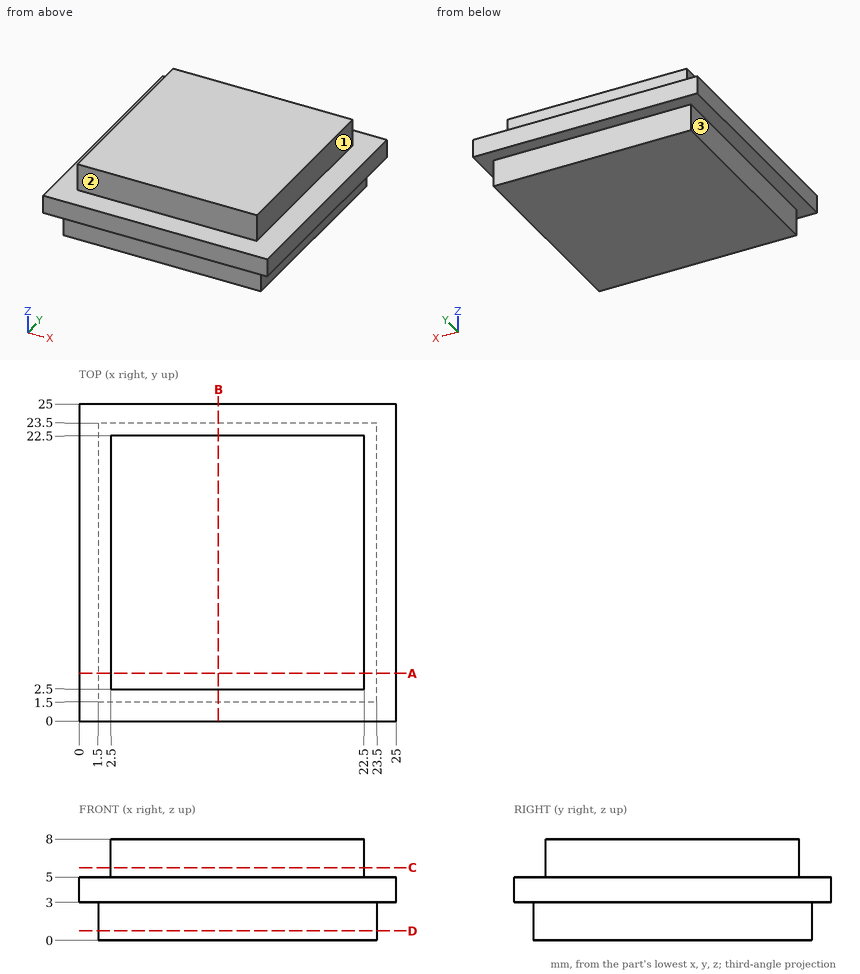
The drawing under review shows one solid part. Ordinate dimensions are in mm from its lowest x, y, z. A direction names the side the tool comes from. Coordinates: 2 decimals unless noted, no trailing zeros. Write each loop counter-clockwise with the first axis right and the second up, starting at its lowest first coordinate (ties: lowest second). Pieces come first, ordered by that corner, then holes. Notation, with made-up numbers: (-25.75, 21) -> (19.25, 21) arc R33 cw to (19.25, 60) -> close; hole circle Ø8 at (5.25, 80). An arc over 180 degrees is marked (long way). Write each question's results on one line, items separated by ' | '. Start each with the question number.
1) Consider section D-D (z = 0.75). Write out the cut boundary in (x, y).
2) Insertion check: pin 1 (0.9 mm diameter, centred on y = 16, z = 2, fed in from -X); pin 2 (0.9 mm diameter, centred on x = 9, z = 2, fed in from -Y); pin 3 (1.5 mm diameter, centred on x = 8, z = 2, fed in from +Y). Each pin has a flat end and moves straight along its axis. Give the tip position at first contact, or say it passes through.
3) Wall thickness on L1, parallel to Y at x = 3.5, z = 7.5; L2, parallel to X at y = 14.5, z = 1: over which ranges is each line inside the solid? List them lowest first. Write a range as [from, to].
4) Consider section C-C (z = 5.75). Write out the cut boundary in (x, y).
5) For the marked faces 1, 2 and 3, list the 3-axis set-ups (+Z, -Z, +X, -X, +Y, -Y) from which the entire face can be reached by the end or side of a thin tool; tool diameter is ignored.
6) Consider section A-A (y = 3.75). Write out the cut boundary in (x, z).
Geometry says:
1) outline: (1.5, 1.5) -> (23.5, 1.5) -> (23.5, 23.5) -> (1.5, 23.5) -> close
2) pin 1: x = 1.5 | pin 2: y = 1.5 | pin 3: y = 23.5
3) L1: [2.5, 22.5] | L2: [1.5, 23.5]
4) outline: (2.5, 2.5) -> (22.5, 2.5) -> (22.5, 22.5) -> (2.5, 22.5) -> close
5) face 1: +Z, +X, +Y, -Y | face 2: +Z, +X, -X, -Y | face 3: -Z, -X, +Y, -Y
6) outline: (0, 3) -> (1.5, 3) -> (1.5, 0) -> (23.5, 0) -> (23.5, 3) -> (25, 3) -> (25, 5) -> (22.5, 5) -> (22.5, 8) -> (2.5, 8) -> (2.5, 5) -> (0, 5) -> close
